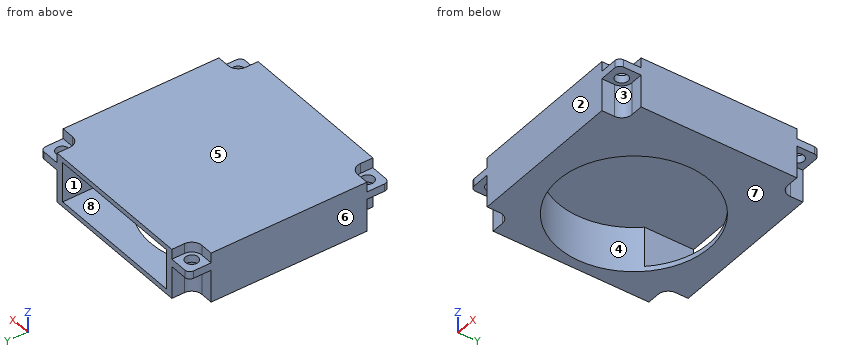
Autodesk Fusion 360 part; units mm, degrees
sketch "Sketch1" plane through (0, 0, 0) normal (0, 0, 1) x (1, 0, 0)
  line L0 (0, 0) -> (20, 0)
  line L1 (20, 0) -> (20, 40)
  line L2 (20, 40) -> (0, 40)
  line L3 (0, 40) -> (0, 0)
  line L4 (0, 0) -> (-20, 0)
  line L5 (-20, 0) -> (-20, 40)
  line L6 (-20, 40) -> (0, 40)
  line L7 (0, 40) -> (0, 0)
  circle A0 centre (-3, 20) radius 15
  circle A1 centre (17.5, 37.5) radius 2
  circle A2 centre (-17.5, 37.5) radius 2
  circle A3 centre (-17.5, 2.5) radius 2
  circle A4 centre (17.5, 2.5) radius 2
  line L8 (17.5, 37.5) -> (17.5, 2.5) construction
  line L9 (17.5, 2.5) -> (-17.5, 2.5) construction
  line L10 (-17.5, 37.5) -> (17.5, 37.5) construction
  circle A5 centre (17.5, 37.5) radius 1.25
  circle A6 centre (-17.5, 37.5) radius 1.25
  circle A7 centre (-17.5, 2.5) radius 1.25
  circle A8 centre (17.5, 2.5) radius 1.25
  line L11 (15.5, 37.5) -> (15.5, 40)
  line L12 (17.5, 35.5) -> (20, 35.5)
  line L13 (17.5, 4.5) -> (20, 4.5)
  line L14 (15.5, 2.5) -> (15.5, 0)
  line L15 (-15.5, 2.5) -> (-15.5, 0)
  line L16 (-17.5, 4.5) -> (-20, 4.5)
  line L17 (-17.5, 35.5) -> (-20, 35.5)
  line L18 (-15.5, 37.5) -> (-15.5, 40)
  dimension "d1" = 40
  dimension "d2" = 40
  dimension "d5" = 30
  dimension "d14" = 17.5
  dimension "d16" = 2.5
  dimension "d17" = 2.5
  dimension "d18" = 2.5
  dimension "d19" = 4
  dimension "d29" = 20
  dimension "d30" = 17
extrude "Extrude1" add sketch "Sketch1" along normal blind 10 contours L0 L1 L2 L3 L7 A0 A1 A4 L11 L12 L13 L14 | L3 L4 L5 L6 L7 A0 A2 A3 L15 L16 L17 L18 | L0 L1 A4 L13 L14 | L3 L7 A0 | L3 L7 A0 | L4 L5 A3 L15 L16 | A4 | A3 | L1 L2 A1 L11 L12 | L5 L6 A2 L17 L18 | A1 | A2 | A5 | A6 | A7 | A8
extrude "Extrude2" cut sketch "Sketch1" along normal blind 9 contours L3 L7 A0 | L3 L7 A0
sketch "Sketch2" plane through (0, 40, 0) normal (0, 1, 0) x (-1, 0, 0)
  line L0 (-20, 0) -> (20, 0)
  line L1 (20, 0) -> (20, 10)
  line L2 (20, 10) -> (-20, 10)
  line L3 (-20, 10) -> (-20, 0)
  line L4 (-14, 1) -> (14, 1)
  line L5 (14, 1) -> (14, 9)
  line L6 (14, 9) -> (-14, 9)
  line L7 (-14, 9) -> (-14, 1)
  line L8 (-14, 1) -> (14, 9) construction
  line L9 (14, 1) -> (-14, 9) construction
  line L10 (0, 5) -> (0, 0) construction
  line L11 (0, 5) -> (-20, 5) construction
  point P0 (0, 5)
  dimension "d9" = 28
  dimension "d10" = 8
extrude "Extrude3" cut sketch "Sketch2" against normal blind 17 contours L4 L5 L6 L7
extrude "Extrude4" cut sketch "Sketch1" along normal blind 6.5 contours L0 L1 A4 L13 L14 | L4 L5 A3 L15 L16 | A4 | A3 | L1 L2 A1 L11 L12 | L5 L6 A2 L17 L18 | A1 | A2 | A5 | A6 | A7 | A8
extrude "Extrude5" cut sketch "Sketch1" along normal blind 44 contours A5 | A6 | A7 | A8
sketch "Sketch3" plane through (0, 0, 10) normal (0, 0, 1) x (1, 0, 0)
  circle A0 centre (-17.5, 37.5) radius 1.25
  circle A1 centre (-17.5, 2.5) radius 1.25
  circle A2 centre (17.5, 37.5) radius 1.25
  circle A3 centre (17.5, 2.5) radius 1.25
  line L0 (-20, 0) -> (20, 0)
  line L1 (20, 0) -> (20, 40)
  line L2 (20, 40) -> (-20, 40)
  line L3 (-20, 40) -> (-20, 0)
  circle A4 centre (-17.5, 37.5) radius 1.25
  arc A5 (-17.5, 35.5) -> (-15.5, 37.5) centre (-17.5, 37.5) ccw
  line L4 (-17.5, 35.5) -> (-20, 35.5)
  line L5 (-20, 35.5) -> (-20, 40)
  line L6 (-20, 40) -> (-15.5, 40)
  line L7 (-15.5, 40) -> (-15.5, 37.5)
  circle A6 centre (17.5, 37.5) radius 1.25
  arc A7 (15.5, 37.5) -> (17.5, 35.5) centre (17.5, 37.5) ccw
  line L8 (15.5, 37.5) -> (15.5, 40)
  line L9 (15.5, 40) -> (20, 40)
  line L10 (20, 40) -> (20, 35.5)
  line L11 (20, 35.5) -> (17.5, 35.5)
  circle A8 centre (-17.5, 2.5) radius 1.25
  arc A9 (-15.5, 2.5) -> (-17.5, 4.5) centre (-17.5, 2.5) ccw
  line L12 (-15.5, 2.5) -> (-15.5, 0)
  line L13 (-15.5, 0) -> (-20, 0)
  line L14 (-20, 0) -> (-20, 4.5)
  line L15 (-20, 4.5) -> (-17.5, 4.5)
  circle A10 centre (17.5, 2.5) radius 1.25
  arc A11 (17.5, 4.5) -> (15.5, 2.5) centre (17.5, 2.5) ccw
  line L16 (17.5, 4.5) -> (20, 4.5)
  line L17 (20, 4.5) -> (20, 0)
  line L18 (20, 0) -> (15.5, 0)
  line L19 (15.5, 0) -> (15.5, 2.5)
extrude "Extrude6" cut sketch "Sketch3" against normal blind 2 contours L0 L3 A9 L12 L13 L14 L15 | L0 L1 A11 L16 L17 L18 L19 | L2 L3 A5 L4 L5 L6 L7 | L1 L2 A7 L8 L9 L10 L11
fillet "Fillet1" radius 1 4 edges at (-20, 0, 7.25) (-20, 40, 7.25) (20, 0, 7.25) (20, 40, 7.25)
equation "d11 = -34.00 mm / 2"
CAD build for the part. Positions are in the model's coordinates, mm. Face numbers are marked on the shaded views. A direction names the side the tool comes from. Coordinates: 2 decimals unless noted, no trailing zeros. Write each loop counter-clockwise with the first axis right and the second up, starting at its lowest first coordinate (ties: lowest second). Pieces come first, ordered by that corner, then holes. Notation, with made-up numbers: (68, -23) -> (117, -23) arc R18 ccw to (117, -6) -> close; hole circle Ø10 at (63.5, -24.75). An arc over 180 degrees is marked (long way). Use CSV: the item, a comma, the result in double quotes. Start each with the question number.
Item 1: Drop flat-ended pins along their axis: P1, Ø0.8, axis at y = 1.5, z = 4, coming from the -X side; P2, Ø3, axis at x = 19.5, z = 2.5, coming from the -Y side; P3, Ø0.6, axis at x = 18.5, z = 9.5, coming from the +Y side; P4, Ø5, axis at x = 13, z = 6, coming from the -Y side. Give the stop position or say it passes through.
Item 2: Tool access for the marked faces 1, 2, 3 and 4: list every direction of +Z, -Z, +X, -X, +Y, -Y with a clear straight run to the whole face (end or side of a thin tool).
Item 3: Wall check: probe 1 along Y at (x, z) = (17.5, 7.55); probe 2 along X at (y, z) = (37.5, 7.35); probe 3 along X at (y, z) = (2.5, 7.4). Give the ranges that are in metal, low to high.
Item 4: Band-saw the part on A-A, the plane x = -3. Write the cut outline in (y, z), plus the area to 3 significant figures.
Item 5: Two-plate mould, pull along Z, no slides. Class the marked faces 5, 6, 7 and 8: +Z half, -Z half, draft (parallel to the pull), parting line (faces both ways), or undercut.
Item 6: Band-saw the part on B-B, the plane z = 3. Write the cut outline in (x, y).
Item 7: Band-saw the part on D-D, the plane x = 6. Write the cut outline in (y, z).
Item 8: Band-saw the part on C-C, the plane y = 20. Write the cut outline in (x, z).
Response values:
1,P1,"stops at x = -15.5"
1,P2,"stops at y = 4.5"
1,P3,"stops at y = 35.5"
1,P4,"stops at y = 0"
2,face 1,"+Y"
2,face 2,"+Z, -Z, +X, -X, -Y"
2,face 3,"-Z, +X, -Y"
2,face 4,"-Z"
3,probe 1,"y = 0 to 1.25, 3.75 to 36.25, 38.75 to 40"
3,probe 2,"x = -20 to -18.75, -16.25 to -14, 14 to 16.25, 18.75 to 20"
3,probe 3,"x = -20 to -18.75, -16.25 to 16.25, 18.75 to 20"
4,outline,"(0, 0) -> (5, 0) -> (5, 9) -> (40, 9) -> (40, 10) -> (0, 10) -> close; (35, 0) -> (40, 0) -> (40, 1) -> (35, 1) -> close"
4,area,"90.0 mm2"
5,face 5,"+Z half"
5,face 6,"draft"
5,face 7,"-Z half"
5,face 8,"undercut"
6,outline,"(-20, 4.5) -> (-17.5, 4.5) arc R2 cw to (-15.5, 2.5) -> (-15.5, 0) -> (15.5, 0) -> (15.5, 2.5) arc R2 cw to (17.5, 4.5) -> (20, 4.5) -> (20, 35.5) -> (17.5, 35.5) arc R2 cw to (15.5, 37.5) -> (15.5, 40) -> (14, 40) -> (14, 23) -> (11.7, 23) arc R15 cw (long way) to (-14, 30.2) -> (-14, 40) -> (-15.5, 40) -> (-15.5, 37.5) arc R2 cw to (-17.5, 35.5) -> (-20, 35.5) -> close"
7,outline,"(0, 0) -> (8, 0) -> (8, 9) -> (40, 9) -> (40, 10) -> (0, 10) -> close; (32, 0) -> (40, 0) -> (40, 1) -> (32, 1) -> close"
8,outline,"(-20, 0) -> (-18, 0) -> (-18, 9) -> (12, 9) -> (12, 0) -> (20, 0) -> (20, 10) -> (-20, 10) -> close"
